Build history of the part. All positions in model axes, mm. A direction names the side the tool comes from. Round coordinates to 2 decimals unless told otherwise and drop trailing zeros. Write each loop counter-clockwise with the first axis right and the second up, starting at its lowest first coordinate (ties: lowest second). Pieces come first, ordered by that corner, then holes. Notation, with made-up numbers: (7.25, -1) -> (30.25, -1) arc R22 ccw to (30.25, 5) -> close; hole circle Ø1 at (62.25, -22.75). An arc over 180 degrees is marked (long way). One line per question, with ' | ' between items.
from build123d import *

# Parameters (mm, degrees)
F0_W          = 316
F0_H          = 16
F1_DEPTH      = 280
F1_DEPTH_BACK = 18
F2_W          = 316
F2_H          = 25
F3_DEPTH      = 16
F4_W          = 316
F4_H          = 18
F5_DEPTH      = 16
F6_W          = 326
F6_H          = 656
F7_DEPTH      = 3
F8_W          = 326
F8_H          = 656
F9_DEPTH      = 3


with BuildPart() as f1:
    # F0 (on Front) → F1 (new body, two sides)
    with BuildSketch(Plane.XZ) as f1_sk:
        Polygon((0, 340), (-175, 340), (-158, 323), (0, 323), (158, 323), (175, 340), align=None)
        Polygon((-158, -323), (-175, -340), (0, -340), (175, -340), (158, -323), (0, -323), align=None)
        Polygon((-158, 323), (-175, 340), (-175, -340), (-158, -323), (-158, -8), (-158, 8), align=None)
        Polygon((175, -340), (175, 340), (158, 323), (158, 8), (158, -8), (158, -323), align=None)
        Rectangle(F0_W, F0_H)
    extrude(amount=F1_DEPTH)
    extrude(f1_sk.sketch, amount=-F1_DEPTH_BACK)

    # F2 (on face) → F3 (cut)
    with BuildSketch(Plane.XY.offset(8)):
        with Locations((0, -267.5)):
            Rectangle(F2_W, F2_H)
    extrude(amount=-F3_DEPTH, mode=Mode.SUBTRACT)

    # F4 (on face) → F5 (cut)
    with BuildSketch(Plane(origin=(0, 0, -8), x_dir=(1, 0, 0), z_dir=(0, 0, -1))):
        with Locations((0, -9)):
            Rectangle(F4_W, F4_H)
    extrude(amount=-F5_DEPTH, mode=Mode.SUBTRACT)

    # F6 (on Front) → F7 (cut)
    with BuildSketch(Plane.XZ):
        Rectangle(F6_W, F6_H)
    extrude(amount=-F7_DEPTH, mode=Mode.SUBTRACT)

    # F8 (on Front) → F9 (join)
    with BuildSketch(Plane.XZ):
        with Locations((0.202316, -2.805007)):
            Rectangle(F8_W, F8_H)
    extrude(amount=-F9_DEPTH)


solid = f1.part
(1) Slice it at A-A (z = -55.5). Write the cut outline in (x, y).
Calculated:
outline: (-175, -280) -> (-158, -280) -> (-158, 0) -> (158, 0) -> (158, -280) -> (175, -280) -> (175, 18) -> (158, 18) -> (158, 3) -> (-158, 3) -> (-158, 18) -> (-175, 18) -> close; hole (-163, 0) -> (-162.8, 0) -> (-162.8, 3) -> (-163, 3) -> close
(2) Slice it at C-C (x = 24). Write the cut outline in (y, z) (3 decimals).
Calculated:
outline: (-280, -340) -> (18, -340) -> (18, -323) -> (3, -323) -> (3, 323) -> (18, 323) -> (18, 340) -> (-280, 340) -> (-280, 323) -> (0, 323) -> (0, 8) -> (-255, 8) -> (-255, -8) -> (0, -8) -> (0, -323) -> (-280, -323) -> close; hole (0, 325.195) -> (3, 325.195) -> (3, 328) -> (0, 328) -> close
(3) Slice it at B-B (y = -137.5). Write the cut outline in (x, z).
Calculated:
outline: (-175, -340) -> (175, -340) -> (175, 340) -> (-175, 340) -> close; hole (-158, -323) -> (158, -323) -> (158, -8) -> (-158, -8) -> close; hole (-158, 8) -> (158, 8) -> (158, 323) -> (-158, 323) -> close
(4) Drop flat-ended pins along their axis: pin 1 (2 mm diameter, centred on x = -76.5, z = 174.5, fed in from -Y); pin 2 (4 mm diameter, centred on x = 14.5, z = -190.5, fed in from +Y); pin 3 (13 mm diameter, centred on x = -26, z = -2.5, fed in from -Y). Give the stop position or say it passes through.
Calculated:
pin 1: y = 0 | pin 2: y = 3 | pin 3: y = -255
(5) 3-axis set-ups, long thin cutter, end or side, ignore diameter. For faces 1 (the flat face through (-2, 3, 5)), 2 (the flat face through (-175, -133, 5)), 3 (the flat face through (-2, 0, -163)): which of +Z, -Z, +X, -X, +Y, -Y reach the whole face in a straight line?
Calculated:
face 1: +Y | face 2: +Z, -Z, -X, +Y, -Y | face 3: -Y
(6) Wall check: line 1 (Z direction, x = 147, y = -149.5); line 2 (X direction, y = -248.5, z = -200.5); line 3 (Z direction, x = -12, y = -267). Give the ranges that are in metal, low to high. Write a range as from..to.
Calculated:
line 1: -340..-323, -8..8, 323..340 | line 2: -175..-158, 158..175 | line 3: -340..-323, 323..340
